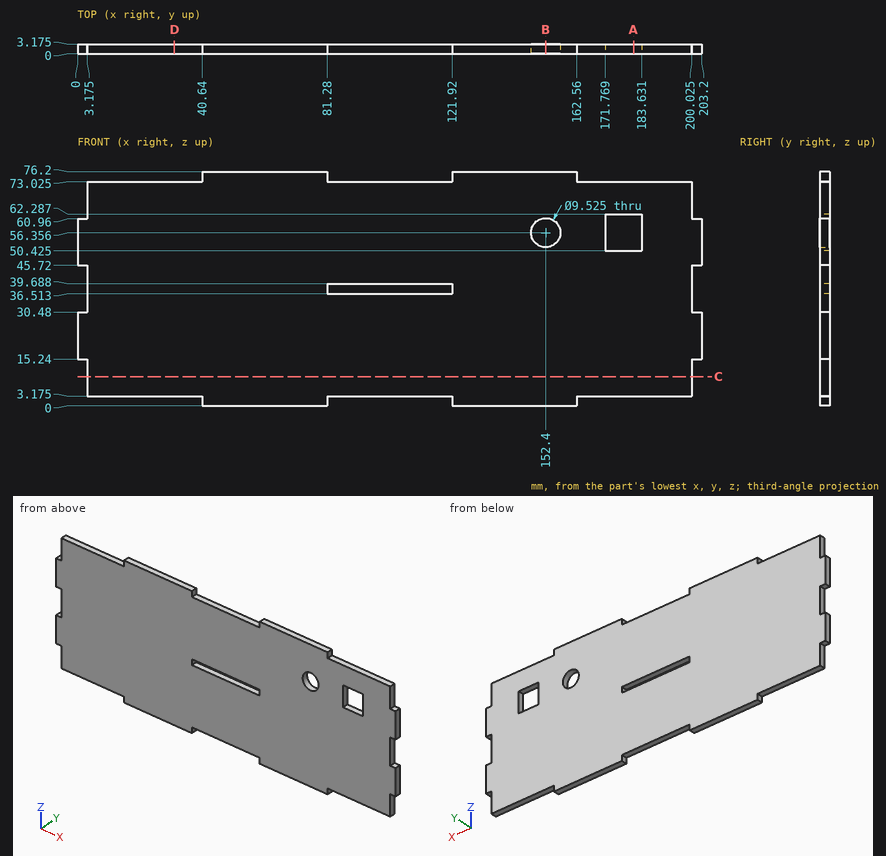
Input: dimensioned drawing with shaded views. Units: mm. Origin: part minimum x, y, z. Round coordinates to 2 decimals unless told otherwise and drop trailing zeros. Loops run counter-clockwise (first coordinate to the right, second up) from the corner with the lowest first, then second, coordinate; pieces in that order, holes last.
1) Material intervals for line 1 (X direction, y = 1.15, z = 38.5) (1 decimal); line 2 (Z direction, x = 152.4, y = 2.25); line 3 (Z direction, x = 105.5, y = 0.5) (1 decimal), sorted ascending.
Ans:
line 1: x = 3.2 to 81.3, 121.9 to 200
line 2: z = 0 to 51.59, 61.12 to 76.2
line 3: z = 3.2 to 36.5, 39.7 to 73
2) Section query D-D on x = 31.5. Return the cut outline in (y, z) (1 decimal), plus the area to 3 significant figures.
Ans:
outline: (0, 3.2) - (3.2, 3.2) - (3.2, 73) - (0, 73) - close
area: 222 mm2
3) Section query B-B on x = 152.4. Return the cut outline in (y, z) (1 decimal), plus the area to 3 significant figures.
Ans:
outline: (0, 0) - (3.2, 0) - (3.2, 51.6) - (0, 51.6) - close; (0, 61.1) - (3.2, 61.1) - (3.2, 76.2) - (0, 76.2) - close
area: 212 mm2
4) Section query C-C on z = 9.5. Return the cut outline in (x, y) (1 decimal).
Ans:
outline: (3.2, 0) - (200, 0) - (200, 3.2) - (3.2, 3.2) - close
5) Section query A-A on x = 181. Return the cut outline in (y, z) (1 decimal), plus the area to 3 significant figures.
Ans:
outline: (0, 3.2) - (3.2, 3.2) - (3.2, 50.4) - (0, 50.4) - close; (0, 62.3) - (3.2, 62.3) - (3.2, 73) - (0, 73) - close
area: 184 mm2
6) Pin query (flat end, axial travel): pin 1 (1 mm diameter, centred on y = 1, z = 2, fed in from +X); pin 2 (1 mm diameter, centred on x = 179.5, y = 1.5, fed in from -Z) (1 decimal); pin 3 (10 mm diameter, centred on x = 29.5, z = 27.5, fed in from -Y); pin 4 (1 mm diameter, centred on x = 2, y = 1.5, fed in from -Z). Return the tip coordinate at first contact, or that it passes through.
Ans:
pin 1: stops at x = 162.56
pin 2: stops at z = 3.2
pin 3: stops at y = 0
pin 4: stops at z = 15.24
